Design review of the part built by this model. Coordinates are the model's own, in mm. A direction names the side the tool comes from. Coordinates: 2 decimals unless noted, no trailing zeros. Loops run counter-clockwise (first coordinate to the right, second up) from the corner with the lowest first, then second, coordinate; pieces in that order, holes last. Notation, with made-up numbers: (36, -9) -> (57, -9) arc R28 cw to (57, 27) -> close; hole circle Ø7 at (58.25, 26). An arc over 180 degrees is marked (long way). Answer as a JSON object with one key per item and string values.
```python
from build123d import *

# Parameters (mm, degrees)
F0_R     = 5.208425
F0_R_2   = 5.19056
F1_DEPTH = 25.4


with BuildPart() as f1:
    # F0 (on Top) → F1 (new body)
    with BuildSketch(Plane.XY):
        with BuildLine():
            Line((-81.381604, 55.626001), (-74.654538, 29.011496))
            ThreePointArc((-74.654538, 29.011496), (-80.618498, 10.506301), (-76.482114, -8.491103))
            Line((-76.482114, -8.491103), (-93.5736, -8.491103))
            Line((-93.5736, -8.491103), (-93.5736, 35.204399))
            Line((-93.5736, 35.204399), (-94.488002, 36.118798))
            Line((-94.488002, 36.118798), (-106.680003, 36.118798))
            Line((-106.680003, 36.118798), (-106.680003, -8.491103))
            Line((-106.680003, -8.491103), (-134.721607, -56.2356))
            Line((-134.721607, -56.2356), (61.874397, -56.2356))
            Line((61.874397, -56.2356), (61.874397, 23.317199))
            Line((61.874397, 23.317199), (36.880802, 23.317199))
            Line((36.880802, 23.317199), (36.727491, 23.317199))
            Line((36.727491, 23.317199), (31.394403, -8.491103))
            Line((31.394403, -8.491103), (-10.081085, -8.491103))
            ThreePointArc((-10.081085, -8.491103), (-5.902864, 9.116501), (-10.484758, 26.623401))
            Line((-10.484758, 26.623401), (-3.657602, 55.626001))
            Line((-3.657602, 55.626001), (-25.71959, 41.685744))
            ThreePointArc((-25.71959, 41.685744), (-40.746905, 45.981971), (-56.217321, 43.758464))
            Line((-56.217321, 43.758464), (-81.381604, 55.626001))
        make_face()
        with Locations((-60.0456, 22.098001)):
            Circle(F0_R, mode=Mode.SUBTRACT)
        with Locations((-31.699203, 23.012402)):
            Circle(F0_R_2, mode=Mode.SUBTRACT)
    extrude(amount=F1_DEPTH)


solid = f1.part
```
1) Add section B-B, the plane z = 4.5. Give the boundary of the cut face in (x, y), and give its area (3 significant figures).
Completed:
{"outline": "(-134.72, -56.24) -> (61.87, -56.24) -> (61.87, 23.32) -> (36.73, 23.32) -> (31.39, -8.49) -> (-10.08, -8.49) arc R37.38 ccw to (-10.48, 26.62) -> (-3.66, 55.63) -> (-25.72, 41.69) arc R37.38 ccw to (-56.22, 43.76) -> (-81.38, 55.63) -> (-74.65, 29.01) arc R37.38 ccw to (-76.48, -8.49) -> (-93.57, -8.49) -> (-93.57, 35.2) -> (-94.49, 36.12) -> (-106.68, 36.12) -> (-106.68, -8.49) -> close; hole circle Ø10.42 at (-60.05, 22.1); hole circle Ø10.38 at (-31.7, 23.01)", "area": "14,000 mm²"}
2) Clearance check with flat-ended pins moving along their axes: pin 1 Ø12.5 at (y, z) = (19, 12.5) entering from -X; pin 2 Ø7.5 at (x, z) = (49, 6.5) entering from +Y; pin 3 Ø3 at (x, z) = (-6, 22.5) entering from +Y; pin 4 Ø8.5 at (x, y) = (-31.7, 23.01) entering from -Z. State where each tip first meets the part, or that it passes through.
Completed:
{"pin 1": "x = -106.68", "pin 2": "y = 23.32", "pin 3": "y = 55.09", "pin 4": "through"}
3) For faces 1 (the flat face through (-68.6, 49.6, 12.5)), 2 (the flat face through (-106.68, 14, 13)), 3 (the flat face through (-78.065, 42.505, 12.522)), list the 3-axis set-ups (+Z, -Z, +X, -X, +Y, -Y) from which the entire face can be reached by the end or side of a thin tool; tool diameter is ignored.
Completed:
{"face 1": "+Z, -Z, +Y", "face 2": "+Z, -Z, -X, +Y", "face 3": "+Z, -Z"}
4) Wall thickness on probe 1 along X at (y, z) = (20, 9.5); probe 2 along Y at (x, z) = (30.5, 2.5); probe 3 along Y at (x, z) = (-98, 10.25): over which ranges is each line inside the solid? List them lowest first.
Completed:
{"probe 1": "-106.68 to -93.57, -78.91 to -64.81, -55.28 to -35.93, -27.47 to -7.65, 36.17 to 61.87", "probe 2": "-56.24 to -8.49", "probe 3": "-56.24 to 36.12"}
5) Add section D-D, the plane y = -13. Give the boundary of the cut face in (x, z).
Completed:
{"outline": "(-109.33, 0) -> (61.87, 0) -> (61.87, 25.4) -> (-109.33, 25.4) -> close"}
6) The part is to be moulded in two halves that separate along Y. For faces 4 (the cylindrical face through (-55.234, 20.103, 12.522)), 5 (the flat face through (34.1, 7.64, 12.52)), 6 (the flat face through (-93.574, 13, 13)), say which applies: pulls with the +Y half, pulls with the -Y half, needs draft (parallel to the pull), parting line crosses it, or undercut.
Completed:
{"face 4": "undercut", "face 5": "pulls with the +Y half", "face 6": "needs draft"}
7) Add section C-C, the plane y = 39. Give the boundary of the cut face in (x, z), and give its area (3 significant figures).
Completed:
{"outline": "(-77.18, 0) -> (-7.57, 0) -> (-7.57, 25.4) -> (-77.18, 25.4) -> close", "area": "1,770 mm²"}
8) Add section A-A, the plane y = 0. Give the boundary of the cut face in (x, z), and give its area (3 significant figures).
Completed:
{"outline": "(-106.68, 0) -> (-93.57, 0) -> (-93.57, 25.4) -> (-106.68, 25.4) -> close; (-79.64, 0) -> (-6.92, 0) -> (-6.92, 25.4) -> (-79.64, 25.4) -> close; (32.82, 0) -> (61.87, 0) -> (61.87, 25.4) -> (32.82, 25.4) -> close", "area": "2,920 mm²"}
